Work out the finished part from the listing and answer in its coordinate system (mm). A direction names the side the tool comes from. Coordinates: 2 decimals unless noted, no trailing zeros. Order: outer loops, then holes, each group sorted by start corner. A loop starts at its lowest first (then second) coordinate and runs counter-clockwise, first axis right, second up. Notation, with made-up numbers: (87, 22) -> (131, 22) arc R17 ccw to (131, 36) -> close; hole circle Ø2 at (-22, 2.5). An arc over 180 degrees is marked (long way). Answer as CSV lines item,"result". Start each with the question number.
Item 1: Straight lines are drawn through the part: L1, parallel to X at y = -10, z = 19.5; L2, parallel to Y at x = -2, z = 77.5; L3, parallel to X at y = 17.65, z = 135. For each, find the intervals that lie inside material, in ascending order.
Item 2: Section A-A (x = 0) is taken. Write down the section's boundary in (y, z).
Item 3: Each of these flat-tipped pins is pushed along its axis until it touches: pin 1 Ø10 at (x, z) = (25.5, 100) entering from -Y; pin 2 Ø10 at (x, z) = (-28.5, 125) entering from -Y; pin 3 Ø1.9 at (x, z) = (0, 135) entering from +Y; pin 4 Ø6 at (x, z) = (-24, 106) entering from -Y. Where does it stop, or does it pass through?
Item 4: Section B-B (z = 15) is taken. Write down the section's boundary in (x, y), then the cut area to 3 significant figures.
Item 5: For a pull along X with two mould halves and no side action, classify faces 1 (the face through (-30.361, 11.495, 73.95)), 2 (the face through (-33.741, 15.185, 73.95)), 3 (the face through (37.5, -6, 74)) as pulls with the +X half, pulls with the -X half, needs draft (parallel to the pull), parting line crosses it, or undercut.
Item 6: Which of the six approach directions +Z, -Z, +X, -X, +Y, -Y give full straight-line access (tool end or side, diameter ignored) to faces 4 (the face through (-35, -18.75, 74)), 5 (the face through (0, 13.75, 74))?
Item 7: Section D-D (x = -31) is taken. Write down the section's boundary in (y, z).
Item 8: Section C-C (x = 23.5) is taken. Write down the section's boundary in (y, z), then the cut area to 3 significant figures.
```python
from build123d import *

# Parameters (mm, degrees)
BOSS_EXTRUDE1_DEPTH = 150
SKETCH2_R           = 1.6
CUT_EXTRUDE1_DEPTH  = 160.099025767
SKETCH4_R           = 7.6
CUT_EXTRUDE2_DEPTH  = 160.099025767


with BuildPart() as part:
    # Sketch1 → Boss-Extrude1 (new body)
    with BuildSketch(Plane(origin=(0, 0, 0), x_dir=(0, 1, 0), z_dir=(0, 0, 1))):
        with BuildLine():
            Line((-18.75, 37.5), (-18.75, 32.5))
            Line((-18.75, 32.5), (6.25, 32.5))
            ThreePointArc((6.25, 32.5), (11.553300859, 30.303300859), (13.75, 25))
            Line((13.75, 25), (13.75, -25))
            ThreePointArc((13.75, -25), (11.553300859, -30.303300859), (6.25, -32.5))
            Line((6.25, -32.5), (-18.75, -32.5))
            Line((-18.75, -32.5), (-18.75, -37.5))
            Line((-18.75, -37.5), (6.25, -37.5))
            ThreePointArc((6.25, -37.5), (15.088834765, -33.838834765), (18.75, -25))
            Line((18.75, -25), (18.75, 25))
            ThreePointArc((18.75, 25), (15.088834765, 33.838834765), (6.25, 37.5))
            Line((6.25, 37.5), (-18.75, 37.5))
        make_face()
    extrude(amount=BOSS_EXTRUDE1_DEPTH)

    # Sketch2 → Cut-Extrude1 (cut, through all)
    with BuildSketch(Plane(origin=(0, 18.75, 0), x_dir=(-1, 0, 0), z_dir=(0, 1, 0))):
        with Locations(Location((0, 135, 0), (0, 0, 90))):
            Circle(SKETCH2_R)
        with Locations(Location((0, 15, 0), (0, 0, 90))):
            Circle(SKETCH2_R)
    extrude(amount=-CUT_EXTRUDE1_DEPTH, mode=Mode.SUBTRACT)

    # Sketch4 → Cut-Extrude2 (cut, through all)
    with BuildSketch(Plane(origin=(0, 18.75, 0), x_dir=(-1, 0, 0), z_dir=(0, 1, 0))):
        with Locations(Location((0, 40, 0), (0, 0, 90))):
            Circle(SKETCH4_R)
    extrude(amount=-CUT_EXTRUDE2_DEPTH, mode=Mode.SUBTRACT)


solid = part.part
```
Checked values:
1,L1,"x = -37.5 to -32.5, 32.5 to 37.5"
1,L2,"y = 13.75 to 18.75"
1,L3,"x = -30.13 to -1.6, 1.6 to 30.13"
2,outline,"(13.75, 0) -> (18.75, 0) -> (18.75, 13.4) -> (13.75, 13.4) -> close; (13.75, 16.6) -> (18.75, 16.6) -> (18.75, 32.4) -> (13.75, 32.4) -> close; (13.75, 47.6) -> (18.75, 47.6) -> (18.75, 133.4) -> (13.75, 133.4) -> close; (13.75, 136.6) -> (18.75, 136.6) -> (18.75, 150) -> (13.75, 150) -> close"
3,pin 1,"stops at y = 11.35"
3,pin 2,"stops at y = -18.75"
3,pin 3,"passes through"
3,pin 4,"stops at y = 13.48"
4,outline,"(-37.5, -18.75) -> (-32.5, -18.75) -> (-32.5, 6.25) arc R7.5 cw to (-25, 13.75) -> (-1.6, 13.75) -> (-1.6, 18.75) -> (-25, 18.75) arc R12.5 ccw to (-37.5, 6.25) -> close; (1.6, 13.75) -> (25, 13.75) arc R7.5 cw to (32.5, 6.25) -> (32.5, -18.75) -> (37.5, -18.75) -> (37.5, 6.25) arc R12.5 ccw to (25, 18.75) -> (1.6, 18.75) -> close"
4,area,"641 mm^2"
5,face 1,"undercut"
5,face 2,"pulls with the -X half"
5,face 3,"pulls with the +X half"
6,face 4,"+Z, -Z, +X, -X, -Y"
6,face 5,"+Z, -Z, -Y"
7,outline,"(10.75, 0) -> (17.22, 0) -> (17.22, 150) -> (10.75, 150) -> close"
8,outline,"(13.75, 0) -> (18.75, 0) -> (18.75, 150) -> (13.75, 150) -> close"
8,area,"750 mm^2"
